Input: part model. Units: mm. Frame: model coordinates. Face numbers are marked on the shaded views. A direction names the side the tool comes from. Round coordinates to 2 decimals unless told otherwise and drop trailing zeros. Loops run counter-clockwise (first coordinate to the right, second up) from the corner with the lowest first, then second, coordinate; pieces in that order, holes last. Notation, with made-up numbers: (-6.75, 0.5) -> (37.25, 0.5) arc R29 cw to (37.25, 31.5) -> close; hole circle Ø3 at (56, 56). An arc over 180 degrees is marked (long way). Answer as a JSON object with one key per item and string values.
```python
from build123d import *

# Parameters (mm, degrees)
SKETCH_1_W          = 50
SKETCH_1_H          = 150
EXTRUDE_1_DEPTH     = 3.5
SKETCH_8_W          = 50
SKETCH_8_H          = 15
SKETCH_8_H_2        = 3.5
SKETCH_8_H_3        = 19.185479081
EXTRUDE_3_DEPTH     = 5
SKETCH_9_R          = 3.302
CUT_EXTRUDE_7_DEPTH = 5
SKETCH_10_R         = 6.731
SKETCH_10_R_2       = 4
SKETCH_10_W         = 15.687252276
SKETCH_10_H         = 63.430283682
CUT_EXTRUDE_8_DEPTH = 10
SKETCH_5_R          = 5.24
CUT_EXTRUDE_9_DEPTH = 10


with BuildPart() as part:
    # 草图1 → 凸台-拉伸1 (new body)
    with BuildSketch(Plane.XY):
        with Locations((1.67844523, -33.188535046)):
            Rectangle(SKETCH_1_W, SKETCH_1_H)
    extrude(amount=EXTRUDE_1_DEPTH)

    # 草图8 → 凸台-拉伸3 (add)
    with BuildSketch(Plane.XZ.offset(108.188535046)):
        with Locations((1.67844523, -7.5)):
            Rectangle(SKETCH_8_W, SKETCH_8_H)
        with Locations((1.67844523, 1.75)):
            Rectangle(SKETCH_8_W, SKETCH_8_H_2)
        with Locations((1.67844523, 13.092739541)):
            Rectangle(SKETCH_8_W, SKETCH_8_H_3)
    extrude(amount=EXTRUDE_3_DEPTH)

    # 草图9 → 切除-拉伸7 (cut)
    with BuildSketch(Plane(origin=(0, -108.188535046, 0), x_dir=(1, 0, 0), z_dir=(0, 1, 0))):
        with Locations(Location((-12.522466831, 7.672144746, 0), (0, 0, 270))):
            Circle(SKETCH_9_R)
        with Locations(Location((17.187336033, 7.672144746, 0), (0, 0, 270))):
            Circle(SKETCH_9_R)
        with Locations(Location((-12.522466831, -12.928520448, 0), (0, 0, 270))):
            Circle(SKETCH_9_R)
        with Locations(Location((17.187336033, -12.928520448, 0), (0, 0, 270))):
            Circle(SKETCH_9_R)
    extrude(amount=-CUT_EXTRUDE_7_DEPTH, mode=Mode.SUBTRACT)

    # 草图10 → 切除-拉伸8 (cut)
    with BuildSketch(Plane.XY.offset(3.5)):
        with Locations((-8.32155477, -91.802996241)):
            Circle(SKETCH_10_R)
        with Locations((-8.32155477, -2.202996241)):
            Circle(SKETCH_10_R)
        with Locations((-8.32155477, 13.397003759)):
            Circle(SKETCH_10_R_2)
        with Locations((-9.087030569, -47.911053293)):
            Rectangle(SKETCH_10_W, SKETCH_10_H)
    extrude(amount=-CUT_EXTRUDE_8_DEPTH, mode=Mode.SUBTRACT)

    # 草图5 → 切除-拉伸9 (cut)
    with BuildSketch(Plane.XY.offset(3.5)):
        with Locations((14.135684743, 13.64917749)):
            Circle(SKETCH_5_R)
        with Locations((14.135684743, -49.462755876)):
            Circle(SKETCH_5_R)
    extrude(amount=-CUT_EXTRUDE_9_DEPTH, mode=Mode.SUBTRACT)


solid = part.part
```
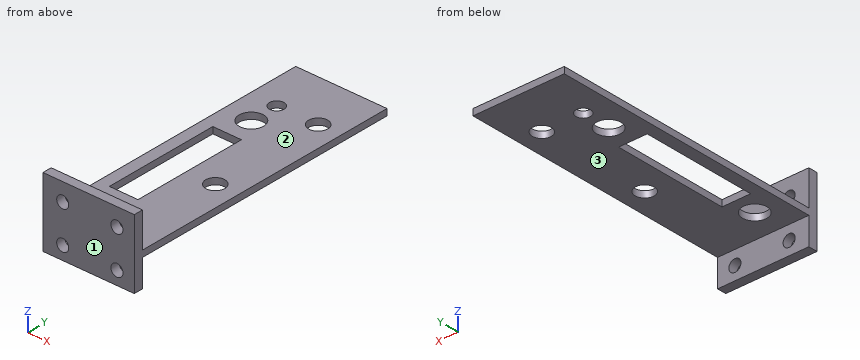
1) Reachability of the marked faces 1, 2 and 3 from +Z, -Z, +X, -X, +Y, -Y: full face, straight path, thin tool, end or side. Return the list, or none.
Output:
{"face 1": "+Z, -Z, +X, -X, -Y", "face 2": "+Z, +X, -X, +Y", "face 3": "-Z, +X, -X, +Y"}
2) Section A-A, the plane y = -64.5. Output: boundary loops of the cut face in (x, z), plus the area to 3 significant figures.
Output:
{"outline": "(-23.32, 0) -> (-16.93, 0) -> (-16.93, 3.5) -> (-23.32, 3.5) -> close; (-1.24, 0) -> (26.68, 0) -> (26.68, 3.5) -> (-1.24, 3.5) -> close", "area": "120 mm^2"}
3) Section D-D, the plane y = 16. Output: boundary loops of the cut face in (x, z).
Output:
{"outline": "(-23.32, 0) -> (-11.36, 0) -> (-11.36, 3.5) -> (-23.32, 3.5) -> close; (-5.28, 0) -> (9.45, 0) -> (9.45, 3.5) -> (-5.28, 3.5) -> close; (18.82, 0) -> (26.68, 0) -> (26.68, 3.5) -> (18.82, 3.5) -> close"}
4) Ray query, probe 1 along Y at (x, z) = (14, 2.5); probe 2 along Y at (x, z) = (15.5, 1); probe 3 along Y at (x, z) = (20.5, -2). Return the intervals inside material, ascending.
Output:
{"probe 1": "y = -113.19 to -54.7, -44.22 to 8.41, 18.89 to 41.81", "probe 2": "y = -113.19 to -54.52, -44.4 to 8.59, 18.71 to 41.81", "probe 3": "y = -113.19 to -108.19"}
5) Contact query for flat-ended pins moving along their axis: P1, Ø6.5, axis at x = -8.32, y = 13.4, coming from the -Z side; P2, Ø17, axis at x = 14.14, y = 13.65, coming from the -Z side; P3, Ø6, axis at x = 4.5, z = 16.5, coming from the +Y side; P4, Ø10, axis at y = -71, z = 6, coming from the +X side. Output: stop coordinate, or through.
Output:
{"P1": "passes through", "P2": "stops at z = 0", "P3": "stops at y = -108.19", "P4": "stops at x = 26.68"}
6) Section C-C, the plane x = -19.5. Output: boundary loops of the cut face in (y, z), plus the area to 3 significant figures.
Output:
{"outline": "(-113.19, -15) -> (-108.19, -15) -> (-108.19, 0) -> (41.81, 0) -> (41.81, 3.5) -> (-108.19, 3.5) -> (-108.19, 22.69) -> (-113.19, 22.69) -> close", "area": "713 mm^2"}
7) Section B-B, the plane z = 13. Output: boundary loops of the cut face in (x, y), plus the area to 3 significant figures.
Output:
{"outline": "(-23.32, -113.19) -> (-15.82, -113.19) -> (-15.82, -108.19) -> (-23.32, -108.19) -> close; (-9.22, -113.19) -> (13.89, -113.19) -> (13.89, -108.19) -> (-9.22, -108.19) -> close; (20.49, -113.19) -> (26.68, -113.19) -> (26.68, -108.19) -> (20.49, -108.19) -> close", "area": "184 mm^2"}
